Here's the drawing with two shaded views (mm, measured from the low corner). I have some questions. Give positions to 0.01 mm unless a question says otherwise; leave off trailing zeros. Loops run counter-clockwise (first coordinate to the right, second up) from the corner with the lowest first, then second, coordinate; pieces in that order, holes last.
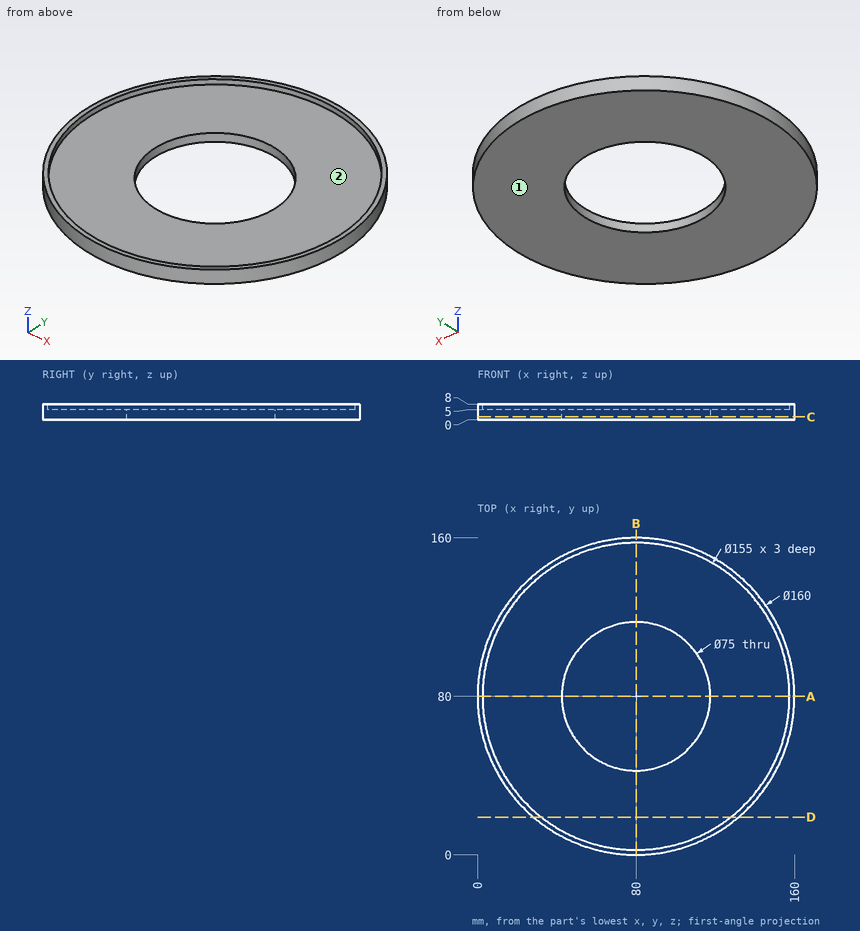
(1) Suppose I cut it at D-D on y = 19. List the corners of the cut face in (x, z) for me, plus the area to 3 significant figures.
Returned:
outline: (28.24, 0) - (131.76, 0) - (131.76, 8) - (127.8, 8) - (127.8, 5) - (32.2, 5) - (32.2, 8) - (28.24, 8) - close
area: 541 mm2
(2) Thinking about a two-plate mould opening in X: for the marked faces 1 and 2, which applies, pulls with the +X half, pulls with the -X half, needs draft (parallel to the pull), parting line crosses it, or undercut?
Returned:
face 1: needs draft
face 2: undercut
(3) Will these pins go through, and if not, where does the flat tip stop? P1, Ø2, axis at x = 117.5, y = 39, coming from the +Z side; P2, Ø2, axis at x = 40, z = 2, coming from the -Y side; P3, Ø1, axis at x = 80, z = 3, coming from the +Y side.
Returned:
P1: stops at z = 5
P2: stops at y = 10.15
P3: stops at y = 160
(4) Suppose I cut it at C-C on z = 1.5. List the corners of the cut face in (x, y) for me.
Returned:
outline: circle Ø160 at (80, 80); hole circle Ø75 at (80, 80)
(5) Please list where these lines run through material, in increasing order: probe 1 along Z at (x, y) = (33.5, 134); probe 2 along Y at (x, z) = (63, 6); probe 3 along X at (y, z) = (76.5, 2.25).
Returned:
probe 1: z = 0 to 5
probe 2: y = 1.83 to 4.39, 155.61 to 158.17
probe 3: x = 0.08 to 42.66, 117.34 to 159.92
(6) Suppose I cut it at A-A on y = 80. List the corners of the cut face in (x, z) for me.
Returned:
outline: (0, 0) - (42.5, 0) - (42.5, 5) - (2.5, 5) - (2.5, 8) - (0, 8) - close; (117.5, 0) - (160, 0) - (160, 8) - (157.5, 8) - (157.5, 5) - (117.5, 5) - close
